```python
from build123d import *

# Parameters (mm, degrees)
SKETCH1_W           = 110
SKETCH1_H           = 60
BOSS_EXTRUDE1_DEPTH = 20
SKETCH3_R           = 5
CUT_EXTRUDE1_DEPTH  = 10
BOSS_EXTRUDE2_DEPTH = 10
SKETCH5_R           = 5
CUT_EXTRUDE2_DEPTH  = 115.127122105


with BuildPart() as part:
    # Sketch1 → Boss-Extrude1 (new body)
    with BuildSketch(Plane(origin=(0, 0, 0), x_dir=(1, 0, 0), z_dir=(0, 1, 0))):
        Rectangle(SKETCH1_W, SKETCH1_H)
    extrude(amount=BOSS_EXTRUDE1_DEPTH)

    # Sketch3 → Cut-Extrude1 (cut)
    with BuildSketch(Plane(origin=(0, 20, 0), x_dir=(1, 0, 0), z_dir=(0, 1, 0))):
        with Locations(Location((-45, 20, 0), (0, 0, 270))):
            Circle(SKETCH3_R)
        with Locations(Location((45, 20, 0), (0, 0, 270))):
            Circle(SKETCH3_R)
        with Locations(Location((45, -20, 0), (0, 0, 270))):
            Circle(SKETCH3_R)
        with Locations(Location((-45, -20, 0), (0, 0, 270))):
            Circle(SKETCH3_R)
    extrude(amount=-CUT_EXTRUDE1_DEPTH, mode=Mode.SUBTRACT)

    # Sketch4 → Boss-Extrude2 (add)
    with BuildSketch(Plane.XY.offset(30)):
        Polygon((-55, 0), (0, -60), (55, 0), (55, 20), (-55, 20), align=None)
    boss_extrude2 = extrude(amount=BOSS_EXTRUDE2_DEPTH)

    # Mirror1: Boss-Extrude2 across plane
    add(boss_extrude2.mirror(Plane.XY))

    # Sketch5 → Cut-Extrude2 (cut, through all)
    with BuildSketch(Plane.XY.offset(40)):
        with Locations((0, -30)):
            Circle(SKETCH5_R)
    extrude(amount=-CUT_EXTRUDE2_DEPTH, mode=Mode.SUBTRACT)


solid = part.part
```
For this review, take the finished solid that the model builds, in its own axes (mm). A direction names the side the tool comes from. Round coordinates to 2 decimals unless told otherwise and drop trailing zeros. Loops run counter-clockwise (first coordinate to the right, second up) from the corner with the lowest first, then second, coordinate; pieces in that order, holes last.
Q1. Insertion check: pin 1 Ø9 at (x, z) = (-45, -20) entering from -Y; pin 2 Ø9 at (x, y) = (0, -30) entering from +Z; pin 3 Ø3 at (x, z) = (-44, -20) entering from +Y; pin 4 Ø1.5 at (y, z) = (-40.5, -29.5) entering from +X. Each pin has a flat end and moves straight along its axis. Give the tip position at first contact, or say it passes through.
Result sheet:
pin 1: stops at y = 0
pin 2: passes through
pin 3: stops at y = 10
pin 4: stops at x = 18.39
Q2. To check wall thickness, follow line 1 along X through (y, z) = (15.25, 20); line 2 along Z through (x, y) = (36, -3); line 3 along X through (y, z) = (12, 18.5). State the ranges of each line that lie inside material, in increasing order.
Result sheet:
line 1: x = -55 to -50, -40 to 40, 50 to 55
line 2: z = -40 to -30, 30 to 40
line 3: x = -55 to -49.77, -40.23 to 40.23, 49.77 to 55
Q3. Mouldability with a two-part tool opening along Y and no side actions: class faces 4 (the face through (-1, 0, 0)), 5 (the face through (-1.08, -34.88, 35.07)), 6 (the face through (49.957, 15.07, 19.349)) as +Y half, -Y half, draft (parallel to the pull), parting line (faces both ways), or undercut.
Result sheet:
face 4: -Y half
face 5: undercut
face 6: draft
Q4. Add section C-C on z = 20. Write out the cut boundary in (x, y), plus the area to 3 significant figures.
Result sheet:
outline: (-55, 0) - (55, 0) - (55, 20) - (50, 20) - (50, 10) - (40, 10) - (40, 20) - (-40, 20) - (-40, 10) - (-50, 10) - (-50, 20) - (-55, 20) - close
area: 2,000 mm2
Q5. Machinability: for faces 1 (the face through (49.957, 15.07, -20.651)), 2 (the face through (-1, -23, -30)), 3 (the face through (27.115, -30.42, -34.93)), which of the approach directions +Z, -Z, +X, -X, +Y, -Y give a long, thin tool a straight path to every point of the face, cutting with its end or side? Answer none if there is none.
Result sheet:
face 1: +Y
face 2: +X, -X, -Y
face 3: +Z, -Z, +X, -Y
Q6. Add section A-A on y = -30. Write out the cut boundary in (x, z).
Result sheet:
outline: (-27.5, -40) - (-5, -40) - (-5, -30) - (-27.5, -30) - close; (-27.5, 30) - (-5, 30) - (-5, 40) - (-27.5, 40) - close; (5, -40) - (27.5, -40) - (27.5, -30) - (5, -30) - close; (5, 30) - (27.5, 30) - (27.5, 40) - (5, 40) - close
Q7. Add section D-D on x = -45. Write out the cut boundary in (y, z).
Result sheet:
outline: (-10.91, -40) - (20, -40) - (20, -25) - (10, -25) - (10, -15) - (20, -15) - (20, 15) - (10, 15) - (10, 25) - (20, 25) - (20, 40) - (-10.91, 40) - (-10.91, 30) - (0, 30) - (0, -30) - (-10.91, -30) - close
Q8. Add section B-B on y = -16. Write out the cut boundary in (x, z), plus the area to 3 significant figures.
Result sheet:
outline: (-40.33, -40) - (40.33, -40) - (40.33, -30) - (-40.33, -30) - close; (-40.33, 30) - (40.33, 30) - (40.33, 40) - (-40.33, 40) - close
area: 1,610 mm2
